Input: part model. Units: mm. Frame: model coordinates. Coordinates: 2 decimals unless noted, no trailing zeros. Loops run counter-clockwise (first coordinate to the right, second up) from the corner with the lowest first, then second, coordinate; pieces in that order, holes last. Notation, with made-up numbers: (83.25, -30) -> (137.25, -30) arc R15 ccw to (137.25, -9) -> close; hole circle Ø9 at (57.25, 34). An arc over 180 degrees is marked (long way). Answer as a JSON object with one key per item and string values.
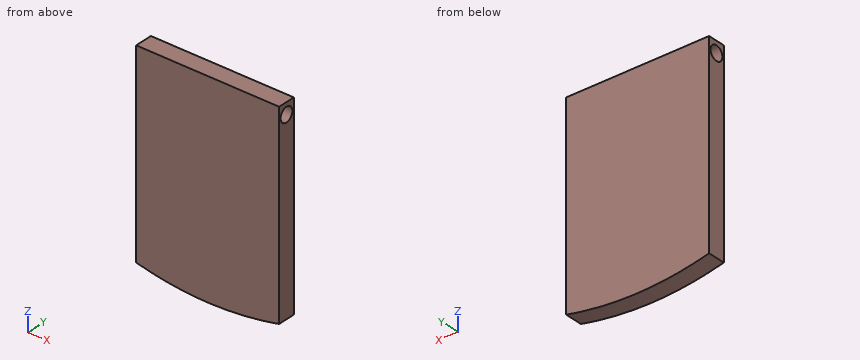
from build123d import *

# Parameters (mm, degrees)
BOSS_EXTRUDE1_DEPTH = 3
SKETCH2_R           = 1.2
CUT_EXTRUDE1_DEPTH  = 7
SKETCH3_R           = 1.2
CUT_EXTRUDE2_DEPTH  = 7
SKETCH4_W           = 24
SKETCH4_H           = 0.6
CUT_EXTRUDE3_DEPTH  = 4.0000001


with BuildPart() as part:
    # Sketch1 → Boss-Extrude1 (new body)
    with BuildSketch(Plane(origin=(0, 0, 0), x_dir=(1, 0, 0), z_dir=(0, 1, 0))):
        with BuildLine():
            Line((0, 0), (24, 0))
            Line((24, 0), (24, 33.6))
            add(Edge.make_bspline(
                [(0, 33.6), (12, 36.4), (24, 33.6)],
                knots=[0, 0, 0, 1, 1, 1], degree=2))
            Line((0, 33.6), (0, 0))
        make_face()
    extrude(amount=BOSS_EXTRUDE1_DEPTH)

    # Sketch2 → Cut-Extrude1 (cut)
    with BuildSketch(Plane(origin=(24, 0, 0), x_dir=(0, 0, -1), z_dir=(1, 0, 0))):
        with Locations((2.5, 1.5)):
            Circle(SKETCH2_R)
    extrude(amount=-CUT_EXTRUDE1_DEPTH, mode=Mode.SUBTRACT)

    # Sketch3 → Cut-Extrude2 (cut)
    with BuildSketch(Plane.ZY):
        with Locations((-2.5, 1.5)):
            Circle(SKETCH3_R)
    extrude(amount=-CUT_EXTRUDE2_DEPTH, mode=Mode.SUBTRACT)

    # Sketch4 → Cut-Extrude3 (cut, through all)
    with BuildSketch(Plane(origin=(0, 3, 0), x_dir=(1, 0, 0), z_dir=(0, 1, 0))):
        with Locations((12, 0.3)):
            Rectangle(SKETCH4_W, SKETCH4_H)
    extrude(amount=-CUT_EXTRUDE3_DEPTH, mode=Mode.SUBTRACT)


solid = part.part
1. Section query A-A (z = -2.5). Return loops of the section in (x, y), plus the area to 3 significant figures.
Reply:
{"outline": "(0, 0) -> (24, 0) -> (24, 0.3) -> (17, 0.3) -> (17, 2.7) -> (24, 2.7) -> (24, 3) -> (0, 3) -> (0, 2.7) -> (7, 2.7) -> (7, 0.3) -> (0, 0.3) -> close", "area": "38.4 mm2"}
2. Line query: line 1 along Y through (x, z) = (20, -2.5); line 2 along X through (y, z) = (1.8, -2.5); line 3 along Z through (x, y) = (2.5, 0.9). Output: solid intervals per line, ascending.
Reply:
{"line 1": "y = 0 to 0.3, 2.7 to 3", "line 2": "x = 7 to 17", "line 3": "z = -34.12 to -3.54, -1.46 to -0.6"}
3. Pin query (flat end, axial travel): P1, Ø0.7, axis at y = 1, z = -2.5, coming from the +X side; P2, Ø0.7, axis at y = 2, z = -2.5, coming from the -X side; P3, Ø3, axis at x = 5.5, z = -20, coming from the -Y side. Return the tip coordinate at first contact, or that it passes through.
Reply:
{"P1": "stops at x = 17", "P2": "stops at x = 7", "P3": "stops at y = 0"}
